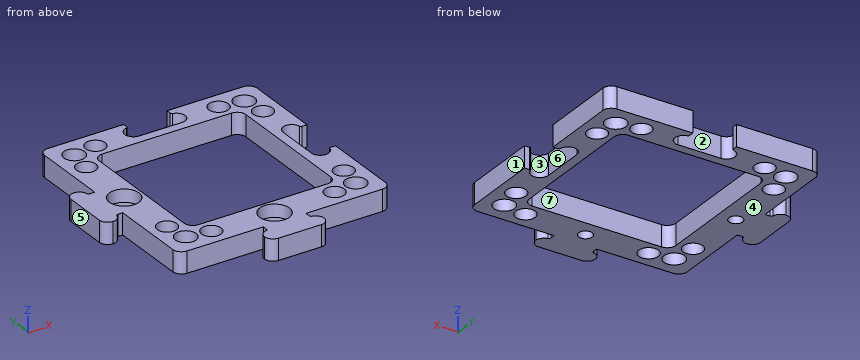
Autodesk Inventor part; units mm, degrees
ref_plane "YZ Plane" through (0, 0, 0) normal (1, 0, 0) x (0, 1, 0)
ref_plane "XZ Plane" through (0, 0, 0) normal (0, 1, 0) x (-1, 0, 0)
ref_plane "XY Plane" through (0, 0, 0) normal (0, 0, 1) x (1, 0, 0)
sketch "Skizze1" plane through (0, 0, 0) normal (0, 0, 1) x (1, 0, 0)
  line L0 (-17.25, 0) -> (-25, 0)
  line L1 (-25, 0) -> (-25, -23)
  line L2 (-23, -25) -> (0, -25)
  line L3 (0, -25) -> (0, -17.25)
  line L4 (-17.25, 0) -> (-17.25, -15.25)
  line L5 (-15.25, -17.25) -> (0, -17.25)
  arc A0 (-25, -23) -> (-23, -25) centre (-23, -23) ccw
  circle A1 centre (-20, -20) radius 2.45
  circle A2 centre (-20.8, -14.5) radius 2.3
  circle A3 centre (-14.5, -20.8) radius 2.3
  arc A4 (-17.25, -15.25) -> (-15.25, -17.25) centre (-15.25, -15.25) ccw
  circle A5 centre (-20, -20) radius 2.45
  circle A6 centre (-14.5, -20.8) radius 2.3
  circle A7 centre (-20.8, -14.5) radius 2.3
  line L6 (-41.8983, 0) -> (36.633, 0) construction
  line L7 (0, -35.5799) -> (0, 35.5799) construction
  point P0 (-25, -25)
  point P1 (-17.25, -17.25)
  dimension "d278" = 25
  dimension "d279" = 25
  dimension "d2" = 7.75
  dimension "d281" = 7.75
  dimension "d282" = 2
  dimension "d283" = 4.9
  dimension "d284" = 20
  dimension "d4" = 20
  dimension "d286" = 4.6
  dimension "d_hole" = 4.6
  dimension "d290" = 20.8
  dimension "d" = 20.8
  dimension "d292" = 2
  dimension "d313" = 6.3
  dimension "d314" = 6.3
  dimension "d330" = 0
  dimension "d331" = 0
  dimension "d332" = 0
extrude "Extrusion1" add sketch "Skizze1" along normal blind 5
mirror "Mirror6" about plane through (-17.25, 0, 0) normal (0, 1, 0) of "Extrusion1"
mirror "Mirror7" about plane through (0, -25, 0) normal (1, 0, 0) of "Extrusion1", "Mirror6"
sketch "Sketch26" plane through (0, 0, 5) normal (0, 0, 1) x (1, 0, 0)
  line L0 (23, 25) -> (-23, 25)
  arc A0 (-23, 25) -> (-25, 23) centre (-23, 23) ccw
  line L1 (-25, -23) -> (-25, 23)
  arc A1 (-25, -23) -> (-23, -25) centre (-23, -23) ccw
  line L2 (-23, -25) -> (23, -25)
  arc A2 (23, -25) -> (25, -23) centre (23, -23) ccw
  line L3 (25, 23) -> (25, -23)
  arc A3 (25, 23) -> (23, 25) centre (23, 23) ccw
  line L4 (15.25, 17.25) -> (-15.25, 17.25)
  arc A4 (17.25, 15.25) -> (15.25, 17.25) centre (15.25, 15.25) ccw
  line L5 (17.25, 15.25) -> (17.25, -15.25)
  arc A5 (15.25, -17.25) -> (17.25, -15.25) centre (15.25, -15.25) ccw
  line L6 (-15.25, -17.25) -> (15.25, -17.25)
  arc A6 (-17.25, -15.25) -> (-15.25, -17.25) centre (-15.25, -15.25) ccw
  line L7 (-17.25, -15.25) -> (-17.25, 15.25)
  arc A7 (-15.25, 17.25) -> (-17.25, 15.25) centre (-15.25, 15.25) ccw
  line L8 (-25, -23) -> (-25, 23)
  line L9 (-28.55, -6.95) -> (-28.55, -6.95)
  line L10 (-30.5, -5) -> (-30.5, 5.1)
  line L11 (-28.55, 7.05) -> (-28.55, 7.05)
  line L12 (-25, 7) -> (-25, -7)
  line L13 (-26.1329, 5) -> (-25, 5)
  line L14 (-25, 5) -> (-25, -5)
  line L15 (-25, -5) -> (-26.1516, -5)
  line L16 (-26.5, -5) -> (-25, 5) construction
  line L17 (-26.5, 5) -> (-25, -5) construction
  arc A8 (-30.5, -5) -> (-28.55, -6.95) centre (-28.55, -5) ccw
  arc A9 (-28.55, -6.95) -> (-26.641, -5.398) centre (-28.55, -5) ccw
  arc A10 (-28.55, 7.05) -> (-30.5, 5.1) centre (-28.55, 5.1) ccw
  arc A11 (-26.6262, 5.4184) -> (-28.55, 7.05) centre (-28.55, 5.1) ccw
  arc A12 (-26.1516, -5) -> (-26.641, -5.398) centre (-26.1516, -5.5) ccw
  arc A13 (-26.6262, 5.4184) -> (-26.1329, 5) centre (-26.1329, 5.5) ccw
  point P0 (0, 0)
  point P1 (-25.75, 0)
  point P2 (-25, 0)
  dimension "d293" = 5.5
  dimension "d294" = 14
  dimension "d296" = 10
  dimension "d297" = 1.5
  dimension "d300" = 1.95
  dimension "d301" = 0.5
  dimension "d357" = 5
extrude "Extrusion13" add sketch "Sketch26" against normal up to surface (5 mm away) contours L1 L15 A12 A9 A8 L10 A10 A11 A13 L13
sketch "Sketch28" plane through (0, 0, 5) normal (0, 0, 1) x (1, 0, 0)
  line L0 (-41.9326, 0) -> (36.8388, 0) construction
  line L1 (23, 25) -> (-23, 25)
  arc A0 (-23, 25) -> (-25, 23) centre (-23, 23) ccw
  line L2 (-25, 5) -> (-25, 23)
  line L3 (-26.1329, 5) -> (-25, 5)
  arc A1 (-26.6262, 5.4184) -> (-26.1329, 5) centre (-26.1329, 5.5) ccw
  arc A2 (-26.6262, 5.4184) -> (-30.5, 5.1) centre (-28.55, 5.1) ccw
  line L4 (-30.5, -5) -> (-30.5, 5.1)
  arc A3 (-30.5, -5) -> (-26.641, -5.398) centre (-28.55, -5) ccw
  arc A4 (-26.1516, -5) -> (-26.641, -5.398) centre (-26.1516, -5.5) ccw
  line L5 (-25, -5) -> (-26.1516, -5)
  line L6 (-25, -23) -> (-25, -5)
  arc A5 (-25, -23) -> (-23, -25) centre (-23, -23) ccw
  line L7 (-23, -25) -> (23, -25)
  arc A6 (23, -25) -> (25, -23) centre (23, -23) ccw
  line L8 (25, 23) -> (25, -23)
  arc A7 (25, 23) -> (23, 25) centre (23, 23) ccw
  circle A8 centre (20, 20) radius 2.45
  circle A9 centre (14.5, 20.8) radius 2.3
  circle A10 centre (20.8, 14.5) radius 2.3
  circle A11 centre (20, -20) radius 2.45
  circle A12 centre (14.5, -20.8) radius 2.3
  circle A13 centre (20.8, -14.5) radius 2.3
  circle A14 centre (-20, 20) radius 2.45
  circle A15 centre (-14.5, 20.8) radius 2.3
  circle A16 centre (-20.8, 14.5) radius 2.3
  circle A17 centre (-20.8, -14.5) radius 2.3
  circle A18 centre (-14.5, -20.8) radius 2.3
  circle A19 centre (-20, -20) radius 2.45
  line L9 (15.25, 17.25) -> (-15.25, 17.25)
  arc A20 (17.25, 15.25) -> (15.25, 17.25) centre (15.25, 15.25) ccw
  line L10 (17.25, 15.25) -> (17.25, -15.25)
  arc A21 (15.25, -17.25) -> (17.25, -15.25) centre (15.25, -15.25) ccw
  line L11 (-15.25, -17.25) -> (15.25, -17.25)
  arc A22 (-17.25, -15.25) -> (-15.25, -17.25) centre (-15.25, -15.25) ccw
  line L12 (-17.25, -15.25) -> (-17.25, 15.25)
  arc A23 (-15.25, 17.25) -> (-17.25, 15.25) centre (-15.25, 15.25) ccw
  line L13 (-25, 5) -> (-24.4142, 5)
  line L14 (-24.4142, 5) -> (-24.4142, -5)
  line L15 (-24.4142, -5) -> (-25, -5)
  line L16 (-25, -5) -> (-25, 5)
  line L17 (-26.1329, 5) -> (-25, 5)
  line L18 (-25, 5) -> (-26.1329, 5)
  line L19 (-30.5, -5) -> (-30.5, 5.1)
  line L20 (-30.5, 5.1) -> (-30.5, -5)
  line L21 (-25, -5) -> (-25, -23)
  line L22 (-25, -5) -> (-26.1516, -5)
  line L23 (-25, -5) -> (-26.1516, -5)
  arc A24 (-26.1516, -5) -> (-26.641, -5.398) centre (-26.1516, -5.5) ccw
  arc A25 (-26.1516, -5) -> (-26.641, -5.398) centre (-26.1516, -5.5) ccw
  arc A26 (-30.5, -5) -> (-26.641, -5.398) centre (-28.55, -5) ccw
  arc A27 (-26.6262, 5.4184) -> (-26.1329, 5) centre (-26.1329, 5.5) ccw
  arc A28 (-26.6262, 5.4184) -> (-30.5, 5.1) centre (-28.55, 5.1) ccw
  arc A29 (-26.6262, 5.4184) -> (-26.1329, 5) centre (-26.1329, 5.5) ccw
  line L24 (25, 5) -> (25.5858, 5)
  line L25 (25.5858, 5) -> (25.5858, -5)
  line L26 (25.5858, -5) -> (25, -5)
  line L27 (25, -5) -> (25, 5)
  line L28 (25, 5) -> (23.8671, 5)
  line L29 (19.5, 5.1) -> (19.5, -5)
  line L30 (25, -5) -> (23.8484, -5)
  arc A30 (23.8484, -5) -> (23.359, -5.398) centre (23.8484, -5.5) ccw
  arc A31 (19.5, -5) -> (23.359, -5.398) centre (21.45, -5) ccw
  arc A32 (23.3738, 5.4184) -> (19.5, 5.1) centre (21.45, 5.1) ccw
  arc A33 (23.3738, 5.4184) -> (23.8671, 5) centre (23.8671, 5.5) ccw
  line L31 (25, 23) -> (25, -23)
  arc A34 (19.4, -5) -> (23.4629, -5.3883) centre (21.45, -5) ccw
  line L32 (19.4, -5) -> (19.4, 5.1)
  arc A35 (23.4725, 5.4347) -> (19.4, 5.1) centre (21.45, 5.1) ccw
  arc A36 (23.4725, 5.4347) -> (23.8671, 5.1) centre (23.8671, 5.5) ccw
  line L33 (23.8671, 5.1) -> (25, 5.1)
  line L34 (25, 5.1) -> (25, -5.1123)
  line L35 (25, -23) -> (25, 23)
  arc A37 (23.8687, -5.1123) -> (23.4629, -5.3883) centre (23.8044, -5.4541) ccw
  line L36 (25, -5.1123) -> (23.8687, -5.1123)
  point P0 (25, -5.1123)
  dimension "d358" = 5.5
  dimension "d359" = 0.1
extrude "Extrusion14" cut sketch "Sketch28" against normal blind 10 contours L8 L28 A33 A32 L29 A31 A30 L30 L36 A37 A34 L32 A35 A36 L33 | L8 L30 A30 A31 L29 A32 A33 L28
pattern_circular "Circular Pattern6" count 2 over 90 about axis through (0, 0, 5) along (0, 0, 1) of "Extrusion14", "Extrusion13"
sketch "Sketch29" plane through (0, 0, 5) normal (0, 0, 1) x (1, 0, 0)
  line L0 (-5.1, 25) -> (-23, 25)
  arc A0 (-23, 25) -> (-25, 23) centre (-23, 23) ccw
  line L1 (-25, 5) -> (-25, 23)
  line L2 (-26.1329, 5) -> (-25, 5)
  arc A1 (-26.6262, 5.4184) -> (-26.1329, 5) centre (-26.1329, 5.5) ccw
  arc A2 (-26.6262, 5.4184) -> (-30.5, 5.1) centre (-28.55, 5.1) ccw
  line L3 (-30.5, -5) -> (-30.5, 5.1)
  arc A3 (-30.5, -5) -> (-26.641, -5.398) centre (-28.55, -5) ccw
  arc A4 (-26.1516, -5) -> (-26.641, -5.398) centre (-26.1516, -5.5) ccw
  line L4 (-25, -5) -> (-26.1516, -5)
  line L5 (-25, -23) -> (-25, -5)
  arc A5 (-25, -23) -> (-23, -25) centre (-23, -23) ccw
  line L6 (-23, -25) -> (-5, -25)
  line L7 (-5, -26.1329) -> (-5, -25)
  arc A6 (-5.4184, -26.6262) -> (-5, -26.1329) centre (-5.5, -26.1329) ccw
  arc A7 (-5.4184, -26.6262) -> (-5.1, -30.5) centre (-5.1, -28.55) ccw
  line L8 (5, -30.5) -> (-5.1, -30.5)
  arc A8 (5, -30.5) -> (5.398, -26.641) centre (5, -28.55) ccw
  arc A9 (5, -26.1516) -> (5.398, -26.641) centre (5.5, -26.1516) ccw
  line L9 (5, -25) -> (5, -26.1516)
  line L10 (5, -25) -> (23, -25)
  arc A10 (23, -25) -> (25, -23) centre (23, -23) ccw
  line L11 (25, -5.1123) -> (25, -23)
  arc A11 (25, 23) -> (23, 25) centre (23, 23) ccw
  line L12 (15.25, 17.25) -> (-15.25, 17.25)
  arc A12 (17.25, 15.25) -> (15.25, 17.25) centre (15.25, 15.25) ccw
  line L13 (17.25, 15.25) -> (17.25, -15.25)
  arc A13 (15.25, -17.25) -> (17.25, -15.25) centre (15.25, -15.25) ccw
  line L14 (-15.25, -17.25) -> (15.25, -17.25)
  arc A14 (-17.25, -15.25) -> (-15.25, -17.25) centre (-15.25, -15.25) ccw
  line L15 (-17.25, -15.25) -> (-17.25, 15.25)
  arc A15 (-15.25, 17.25) -> (-17.25, 15.25) centre (-15.25, 15.25) ccw
  circle A16 centre (-21.36, 0) radius 3.89
  circle A17 centre (0, -21.36) radius 2.9259
  line L16 (-41.8983, 0) -> (36.633, 0) construction
  line L17 (0, -41.8983) -> (0, 36.633) construction
  line L18 (5.1123, 25) -> (5.1123, 23.8687)
  arc A18 (5.1123, 23.8687) -> (5.3883, 23.4629) centre (5.4541, 23.8044) ccw
  arc A19 (5, 19.4) -> (5.3883, 23.4629) centre (5, 21.45) ccw
  line L19 (5, 19.4) -> (-5.1, 19.4)
  arc A20 (-5.4347, 23.4725) -> (-5.1, 19.4) centre (-5.1, 21.45) ccw
  arc A21 (-5.4347, 23.4725) -> (-5.1, 23.8671) centre (-5.5, 23.8671) ccw
  line L20 (-5.1, 23.8671) -> (-5.1, 25)
  line L21 (25, -5.1123) -> (23.8687, -5.1123)
  arc A22 (23.8687, -5.1123) -> (23.4629, -5.3883) centre (23.8044, -5.4541) ccw
  arc A23 (19.4, -5) -> (23.4629, -5.3883) centre (21.45, -5) ccw
  line L22 (19.4, -5) -> (19.4, 5.1)
  arc A24 (23.4725, 5.4347) -> (19.4, 5.1) centre (21.45, 5.1) ccw
  arc A25 (23.4725, 5.4347) -> (23.8671, 5.1) centre (23.8671, 5.5) ccw
  line L23 (23.8671, 5.1) -> (25, 5.1)
  line L24 (25, 23) -> (25, 5.1)
  line L25 (23, 25) -> (5.1123, 25)
  point P0 (0, 0)
  dimension "d319" = 7.78
  dimension "d320" = 4.11
  dimension "d322" = 4.11
hole "Hole7" at (-21.36, 0, 5) at (0, -21.36, 5) direction (0, 0, -1) diameter 3.2 end through all counterbore diameter 7 counterbore depth 3
equation "\"d_i\" = 40"
equation "\"d_o\" = 40"
equation "\"d_part\" = 50"
equation "\"d6\" = 0"
equation "\"d7\" = 0"
equation "\"d8\" = 0"
equation "\"d9\" = 0"
equation "\"d13\" = 0"
equation "\"d14\" = 0"
equation "\"d20\" = 0"
equation "\"d21\" = 0"
equation "\"d22\" = 0"
equation "\"d23\" = 0"
equation "\"d24\" = 0"
equation "\"d25\" = 3"
equation "\"d26\" = 0"
equation "\"d27\" = 0"
equation "\"d28\" = 0"
equation "\"d29\" = 0"
equation "\"d30\" = 0"
equation "\"d31\" = 0"
equation "\"d32\" = 0"
equation "\"d33\" = 0"
equation "\"d34\" = 0"
equation "\"d46\" = 0"
equation "\"d47\" = 0"
equation "\"d48\" = 0"
equation "\"d50\" = 0"
equation "\"d51\" = 0"
equation "\"d52\" = 0"
equation "\"d53\" = 0"
equation "\"d54\" = 0"
equation "\"d55\" = 0"
equation "\"d56\" = 0"
equation "\"d57\" = 0"
equation "\"d58\" = 0"
equation "\"d59\" = 0"
equation "\"magnet_offset\" = 0"
equation "\"screw_offset\" = 0"
equation "\"mal_puzzle_offset\" = 0"
equation "\"fem_puzzle_offset\" = 0"
properties part number "10_Base_puzzle_v3"
Build history of the part. All positions in model axes, mm. Face numbers are marked on the shaded views. A direction names the side the tool comes from. Coordinates: 2 decimals unless noted, no trailing zeros. Order: outer loops, then holes, each group sorted by start corner. A loop starts at its lowest first (then second) coordinate and runs counter-clockwise, first axis right, second up. Notation, with made-up numbers: M 47.25,86.25 L 73.25,86.25 A22 ccw 73.25,110.25 Z; hole C 57,-34 d2. An arc over 180 degrees is marked long. One line per question, with ' | ' between items. Start each with the question number.
Q1. 3-axis set-ups, long thin cutter, end or side, ignore diameter. For the marked faces 5, 6 and 7: which of +Z, -Z, +X, -X, +Y, -Y reach the whole face in a straight line?
Q2. Probe L1, parallel to Y at x = -20, z = 2.3; L2, parallel to Y at x = 20.8, z = 2.7; L3, parallel to X at y = 6, z = 3.3. List the from-to ranges inside material, lowest first. Write a range as from..to.
Q3. Saw through at C-C (x = 20.8). List the corners of the cut face in (y, z), then the cut area to 3 significant figures.
Q4. Flat gauge pins, fed straight in: pin 1 Ø1.2 at (x, z) = (24, 3) entering from +Y; pin 2 Ø1.5 at (y, z) = (-23, 3) entering from -X. Where does each tip first touch, or does it go through?
Q5. Two-plate mould, pull along X, no slides. Class the marked faces 1, 2, 3 and 4: +X half, -X half, draft (parallel to the pull), parting line (faces both ways), or undercut.
Q6. Saw through at D-D (x = -16). List the corners of the cut face in (y, z), then the cut area to 3 significant figures.
Q7. Saw through at B-B (y = -14.5). List the corners of the cut face in (x, z), then the cut area to 3 significant figures.
Q8. Saw through at A-A (x = 10.5). List the corners of the cut face in (y, z), then the cut area to 3 significant figures.
Check values:
1) face 5: +Z, -Z, -X, +Y, -Y | face 6: +Z, -Z, +X | face 7: +Z, -Z
2) L1: y = -25..-22.45, -17.55..-16.66, -12.34..-3.22, 3.22..12.34, 16.66..17.55, 22.45..25 | L2: y = -25..-22.32, -17.68..-16.8, -12.2..-6.94, 7.04..12.2, 16.8..17.68, 22.32..25 | L3: x = -30.28..-26.82, -25..-17.25, 17.25..19.61, 23.29..25
3) outline: M -25,0 L -22.32,0 L -22.32,5 L -25,5 Z; M -17.68,0 L -16.8,0 L -16.8,5 L -17.68,5 Z; M -12.2,0 L -6.94,0 L -6.94,5 L -12.2,5 Z; M 7.04,0 L 12.2,0 L 12.2,5 L 7.04,5 Z; M 16.8,0 L 17.68,0 L 17.68,5 L 16.8,5 Z; M 22.32,0 L 25,0 L 25,5 L 22.32,5 Z | area: 87.7 mm2
4) pin 1: stops at y = 24.96 | pin 2: stops at x = -25
5) face 1: +X half | face 2: undercut | face 3: undercut | face 4: draft
6) outline: M -25,0 L -22.54,0 L -22.54,5 L -25,5 Z; M -19.06,0 L -17.1,0 L -17.1,5 L -19.06,5 Z; M 17.1,0 L 19.06,0 L 19.06,5 L 17.1,5 Z; M 22.54,0 L 25,0 L 25,5 L 22.54,5 Z | area: 44.1 mm2
7) outline: M -25,0 L -23.1,0 L -23.1,5 L -25,5 Z; M -18.5,0 L -17.25,0 L -17.25,5 L -18.5,5 Z; M 17.25,0 L 18.5,0 L 18.5,5 L 17.25,5 Z; M 23.1,0 L 25,0 L 25,5 L 23.1,5 Z | area: 31.5 mm2
8) outline: M -25,0 L -17.25,0 L -17.25,5 L -25,5 Z; M 17.25,0 L 25,0 L 25,5 L 17.25,5 Z | area: 77.5 mm2
